Answer from the drawing. Dimensions are ordinates in mm from the lowest x, y and z of the part. A direction names the side the tool comes from. Coordinates: 2 decimals unless noted, no trailing zeros. Order: outer loops, then holes, each group sorted by start corner. A loop starts at its lowest first (then second) coordinate and runs counter-clockwise, first axis right, second up. Notation, with made-up numbers: (71.5, 69) - (120.5, 69) arc R15 cw to (120.5, 95) - close; hole circle Ø4 at (63, 67.25). An arc over 180 degrees is marked (long way). Answer as a JSON object with one key per item and string values. Group by question number.
1) Each of these flat-tipped pins is pushed along its axis until it touches: P1, Ø3, axis at x = 17.5, z = 6, coming from the -Y side; P2, Ø5.5, axis at x = 30, z = 15, coming from the -Y side. Where does it stop, or does it pass through?
2) Find the intervals of material crossed by line 1 along X through (y, z) = (4.95, 15); line 2 along X through (y, z) = (0.5, 12.75); line 3 along Z through (x, y) = (30, 6.55), in increasing order.
3) Section A-A (x = 30) is taken. Give the vertices of the cut face in (y, z).
4) Section B-B (z = 15) is taken. Give the vertices of the cut face in (x, y), plus the area to 3 significant figures.
5) Section C-C (z = 8) is taken. Give the vertices of the cut face in (x, y).
6) The mould has two halves that part along Z. Classify the marked faces 1, 2, 3 and 4: released by +Z, released by -Z, zero draft, split by the parting line, or undercut.
7) Section D-D (x = 47.5) is taken. Give the vertices of the cut face in (y, z).
8) A tool of negligible diameter and unlimited length cuts with its end or side. For the marked faces 5 and 6, from which of +Z, -Z, +X, -X, +Y, -Y can it reach the whole face along a straight path? Write none if from no direction.
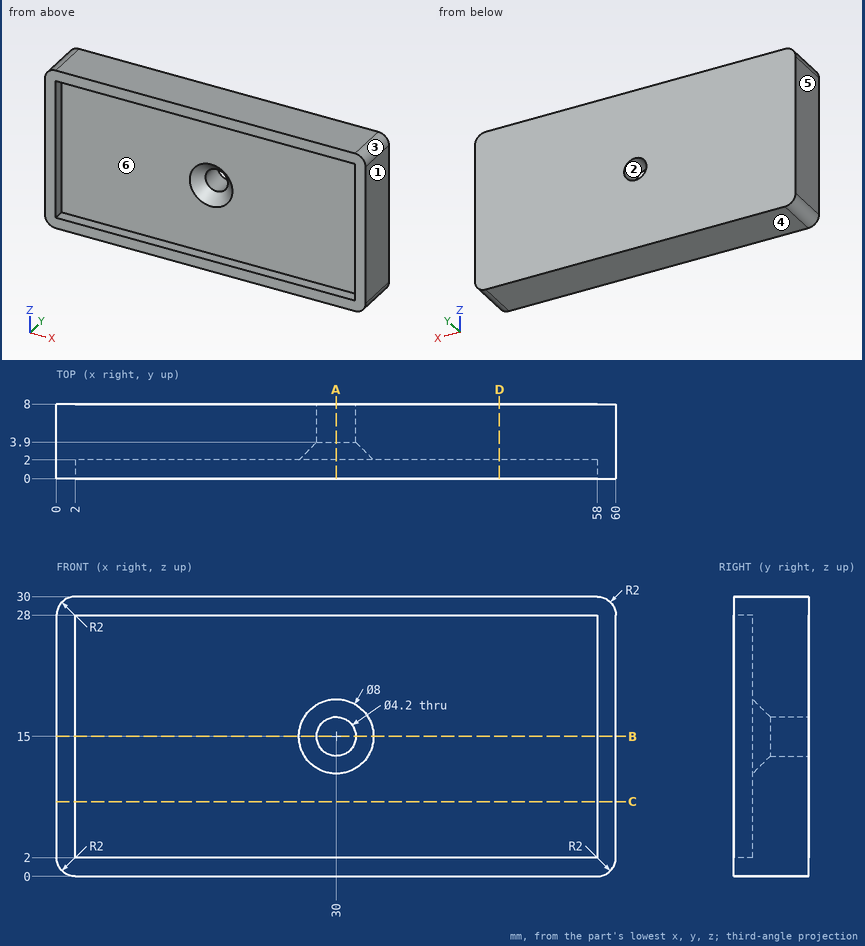
Report:
{
 "1": {"P1": "stops at y = 2", "P2": "stops at y = 3.25"},
 "2": {"line 1": "x = 0 to 27.9, 32.1 to 60", "line 2": "x = 0 to 2, 58 to 60", "line 3": "z = 0 to 12.9, 17.1 to 30"},
 "3": {"outline": "(0, 0) - (8, 0) - (8, 12.9) - (3.9, 12.9) - (2, 11) - (2, 2) - (0, 2) - close; (0, 28) - (2, 28) - (2, 19) - (3.9, 17.1) - (8, 17.1) - (8, 30) - (0, 30) - close"},
 "4": {"outline": "(0, 0) - (2, 0) - (2, 2) - (26, 2) - (27.9, 3.9) - (27.9, 8) - (0, 8) - close; (32.1, 3.9) - (34, 2) - (58, 2) - (58, 0) - (60, 0) - (60, 8) - (32.1, 8) - close", "area": "339 mm²"},
 "5": {"outline": "(0, 0) - (2, 0) - (2, 2) - (58, 2) - (58, 0) - (60, 0) - (60, 8) - (0, 8) - close"},
 "6": {"face 1": "zero draft", "face 2": "undercut", "face 3": "released by +Z", "face 4": "released by -Z"},
 "7": {"outline": "(0, 0) - (8, 0) - (8, 30) - (0, 30) - (0, 28) - (2, 28) - (2, 2) - (0, 2) - close"},
 "8": {"face 5": "+Z, -Z, -X, +Y, -Y", "face 6": "-Y"}
}
